from build123d import *

# Parameters (mm, degrees)
F2_R     = 1
F3_SIZE  = 1.5
F5_DEPTH = 7


with BuildPart() as f1:
    # F0 (on Top) → F1 (revolve)
    with BuildSketch(Plane.XY):
        Polygon((-30.745121, 9), (-30.745121, 0), (21.254879, 0), (21.254879, 6), (-18.745121, 6), (-18.745121, 9), align=None)
    revolve(axis=Axis((0.541581, 0, 0), (1, 0, 0)))

    # F2
    f2_edges = [f1.edges().sort_by_distance(p)[0] for p in [
        (-30.745121, -9, 0),
    ]]
    fillet(f2_edges, radius=F2_R)

    # F3
    f3_edges = [f1.edges().sort_by_distance(p)[0] for p in [
        (21.254879, -6, 0),
    ]]
    chamfer(f3_edges, length=F3_SIZE)

    # F4 (on face) → F5 (cut)
    with BuildSketch(Plane(origin=(-30.745121, 0, 0), x_dir=(0, -1, 0), z_dir=(-1, 0, 0))):
        Polygon((5, -2.886751), (5, 0), (5, 2.886751), (0, 5.773503), (-5, 2.886751), (-5, 0), (-5, -2.886751), (0, -5.773503), align=None)
    extrude(amount=-F5_DEPTH, mode=Mode.SUBTRACT)

    # F6 (on Front) → F7 (revolve, cut)
    with BuildSketch(Plane.XZ):
        Polygon((-30.245121, 5.273503), (-30.745121, 5.773503), (-30.745121, 0), (-30.245121, 0), align=None)
    revolve(axis=Axis((0.541581, 0, 0), (1, 0, 0)), mode=Mode.SUBTRACT)


with BuildPart() as f8_1:
    # F8: copy of F1
    add(f1.part)


solid = f1.part
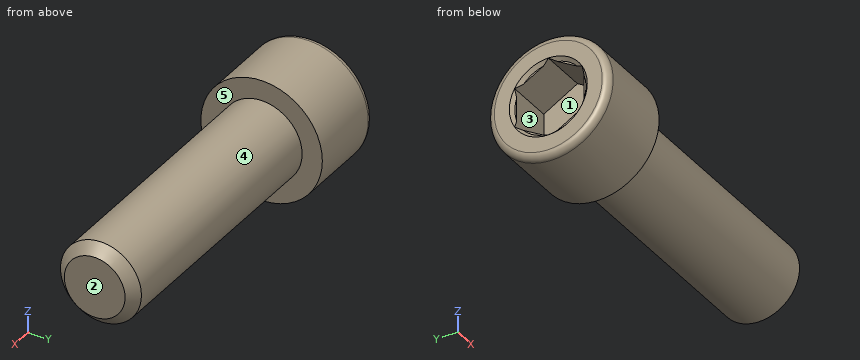
Work out the finished part from the listing and answer in its coordinate system (mm). Face numbers are marked on the shaded views. A direction names the side the tool comes from. Round coordinates to 2 decimals unless told otherwise and drop trailing zeros. Loops run counter-clockwise (first coordinate to the right, second up) from the corner with the lowest first, then second, coordinate; pieces in that order, holes last. Notation, with made-up numbers: (1, -37.75) - (17, -37.75) arc R23 cw to (17, -19.75) - close; hole circle Ø10 at (59.5, 72). An arc over 180 degrees is marked (long way). Use one line per item in the form item = value. Start each with the question number.
(1) Find section C-C on x = -14. Determine the outline of the cut face in (y, z).
(2) Flat-ended cylindrical pins translate along their axes: P1, Ø5, axis at y = 1.5, z = -1.5, coming from the -X side; P2, Ø0.8, axis at y = -3, z = 4, coming from the -X side; P3, Ø1.5, axis at x = 2.5, y = -4, coming from the +Z side. Find the tip coordinate at first contact, or state that the pin passes through.
(3) Determine the mould class of the marked faces 3, 4 and 5 for opening direction Z: +Z half, -Z half, draft (parallel to the pull), parting line (faces both ways), or undercut.
(4) Find section B-B on x = -21.5. Determine the outline of the cut face in (y, z), and give its area (3 significant figures).
(5) Which of the six approach directions +Z, -Z, +X, -X, +Y, -Y give full straight-line access (tool end or side, diameter ignored) to the marked faces 1 and 2?
(6) Consider line 1 (X direction, y = 5.5, z = -5.5); line 2 (X direction, y = -0.25, z = -3.5); line 3 (Y direction, x = -2, z = -0.25). Determine where each line is inside the solid, lowest interval first.
(7) Find section A-A on z = 0. Determine the outline of the cut face in (x, y).
Answer list:
q1.outline = circle Ø12 at (0, 0)
q2.P1 = -23.75
q2.P2 = -30.37
q2.P3 = 5.04
q3.face_3 = undercut
q3.face_4 = parting line
q3.face_5 = draft
q4.outline = circle Ø18 at (0, 0)
q4.area = 254 mm^2
q5.face_1 = -X
q5.face_2 = +Z, -Z, +X, +Y, -Y
q6.line_1 = -30.75 to -18.75
q6.line_2 = -23.75 to 21.25
q6.line_3 = -5.99 to 5.99
q7.outline = (-30.75, -8) arc R1 ccw to (-29.75, -9) - (-18.75, -9) - (-18.75, -6) - (19.75, -6) - (21.25, -4.5) - (21.25, 4.5) - (19.75, 6) - (-18.75, 6) - (-18.75, 9) - (-29.75, 9) arc R1 ccw to (-30.75, 8) - (-30.75, 5.77) - (-30.25, 5.27) - (-30.25, 5) - (-23.75, 5) - (-23.75, -5) - (-30.25, -5) - (-30.25, -5.27) - (-30.75, -5.77) - close
